Design review of the part shown in the three views and the two pictorial views. Dimensions are in mm from the part's minimum x, y and z. Give positions to 0.01 mm unless a question says otherwise; leave off trailing zeros. Order: outer loops, then holes, each group sorted by start corner. A loop starts at its lowest first (then second) coordinate and runs counter-clockwise, first axis right, second up.
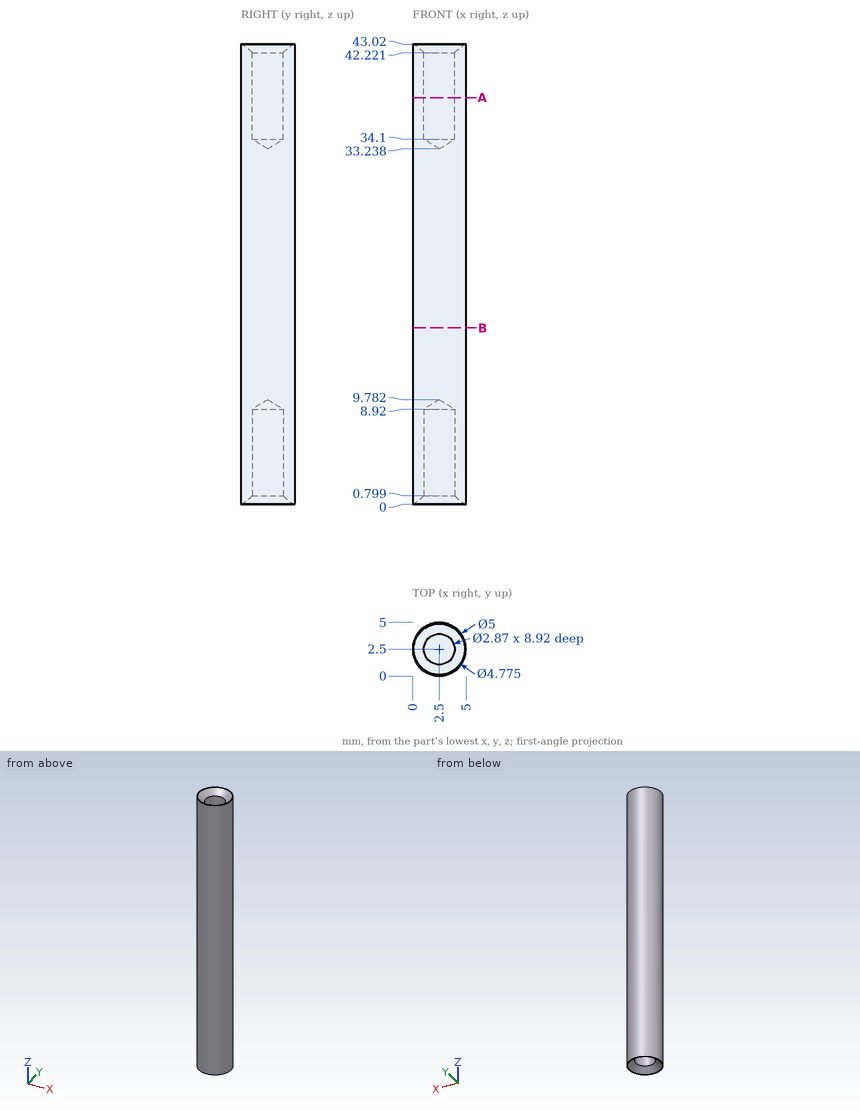
Item 1: Take a section at B-B (z = 16.5). Give the boundary of the cut face in (x, y).
Values found:
outline: circle Ø5 at (2.5, 2.5)
Item 2: For line 1 (Y direction, x = 2.5, z = 37.25) (1 decimal); line 2 (Y direction, x = 3.25, z = 19) (1 decimal); line 3 (Y direction, x = 4.55, z = 35), list the stretches that pass through material, from the lowest coordinate up.
Values found:
line 1: y = 0 to 1.1, 3.9 to 5
line 2: y = 0.1 to 4.9
line 3: y = 1.07 to 3.93
Item 3: Take a section at A-A (z = 38). Give the boundary of the cut face in (x, y) (1 decimal).
Values found:
outline: circle Ø5 at (2.5, 2.5); hole circle Ø2.9 at (2.5, 2.5)
Item 4: Clearance check with flat-ended pins moving along their axes: pin 1 Ø2 at (y, z) = (4, 34) entering from +X; pin 2 Ø2 at (y, z) = (4.5, 27) entering from +X; pin 3 Ø2 at (x, z) = (4, 25) entering from +Y. State where each tip first meets the part, or that it passes through.
Values found:
pin 1: stops at x = 4.95
pin 2: stops at x = 4.79
pin 3: stops at y = 4.95
